```python
from build123d import *

# Parameters (mm, degrees)
SKETCH1_R                         = 5
BOSS_EXTRUDE1_DEPTH               = 2
SKETCH2_W                         = 2
SKETCH2_H                         = 4
CUT_EXTRUDE_THIN1_DEPTH           = 2
CUT_EXTRUDE_THIN1_DRAFT           = -17
SKETCH2_W_2                       = 4
SKETCH2_H_2                       = 2
CUT_EXTRUDE_THIN1_PROFILE_2_DEPTH = 2
CUT_EXTRUDE_THIN1_PROFILE_2_DRAFT = -17
SKETCH3_R                         = 2
BOSS_EXTRUDE2_DEPTH               = 40


with BuildPart() as part:
    # Sketch1 → Boss-Extrude1 (new body)
    with BuildSketch(Plane(origin=(0, 0, 0), x_dir=(1, 0, 0), z_dir=(0, 1, 0))):
        with Locations(Location((0, 0, 0), (0, 0, 270))):
            Circle(SKETCH1_R)
    extrude(amount=BOSS_EXTRUDE1_DEPTH)


with BuildPart() as cut_extrude_thin1_tool:
    # Sketch2 → Cut-Extrude-Thin1 (with draft: the straight prism first)
    with BuildSketch(Plane(origin=(0, 2, 0), x_dir=(1, 0, 0), z_dir=(0, 1, 0))):
        Rectangle(SKETCH2_W, SKETCH2_H)
    extrude(amount=-CUT_EXTRUDE_THIN1_DEPTH)
    # Cut-Extrude-Thin1: the draft: its side faces are tilted about the plane it starts from
    cut_extrude_thin1_sides = [cut_extrude_thin1_tool.faces().sort_by_distance(p)[0] for p in [
        (1, 1, 0),
        (0, 1, -2),
        (-1, 1, 0),
        (0, 1, 2),
    ]]
    draft(cut_extrude_thin1_sides, Plane(origin=(0, 2, 0), x_dir=(1, 0, 0), z_dir=(0, 1, 0)), CUT_EXTRUDE_THIN1_DRAFT)


with BuildPart() as part_1:
    add(part.part)

    # Cut-Extrude-Thin1: cut by cut_extrude_thin1_tool
    add(cut_extrude_thin1_tool.part, mode=Mode.SUBTRACT)


with BuildPart() as cut_extrude_thin1_profile_2_tool:
    # Sketch2 → Cut-Extrude-Thin1 profile 2 (with draft: the straight prism first)
    with BuildSketch(Plane(origin=(0, 2, 0), x_dir=(1, 0, 0), z_dir=(0, 1, 0))):
        Rectangle(SKETCH2_W_2, SKETCH2_H_2)
    extrude(amount=-CUT_EXTRUDE_THIN1_PROFILE_2_DEPTH)
    # Cut-Extrude-Thin1 profile 2: the draft: its side faces are tilted about the plane it starts from
    cut_extrude_thin1_profile_2_sides = [cut_extrude_thin1_profile_2_tool.faces().sort_by_distance(p)[0] for p in [
        (0, 1, 1),
        (2, 1, 0),
        (0, 1, -1),
        (-2, 1, 0),
    ]]
    draft(cut_extrude_thin1_profile_2_sides, Plane(origin=(0, 2, 0), x_dir=(1, 0, 0), z_dir=(0, 1, 0)), CUT_EXTRUDE_THIN1_PROFILE_2_DRAFT)


with BuildPart() as part_2:
    add(part_1.part)

    # Cut-Extrude-Thin1 profile 2: cut by cut_extrude_thin1_profile_2_tool
    add(cut_extrude_thin1_profile_2_tool.part, mode=Mode.SUBTRACT)

    # Sketch3 → Boss-Extrude2 (add)
    with BuildSketch(Plane.XZ):
        with Locations(Location((0, 0, 0), (0, 0, 90))):
            Circle(SKETCH3_R)
    extrude(amount=BOSS_EXTRUDE2_DEPTH)


solid = part_2.part
```
The model under review builds one solid part; all positions refer to its coordinate system, in mm. A direction names the side the tool comes from. Give positions to 0.01 mm unless a question says otherwise; leave off trailing zeros. Write each loop counter-clockwise with the first axis right and the second up, starting at its lowest first coordinate (ties: lowest second). Pieces come first, ordered by that corner, then holes. Notation, with made-up numbers: (12.25, -28.5) - (64.25, -28.5) arc R11 cw to (64.25, -20.5) - close; hole circle Ø3 at (-15, 65.25). An arc over 180 degrees is marked (long way). Answer in a Markdown table with one row per item. Add a question column.
1. Wall thickness on line 1 along Y through (x, z) = (1.5, -4.5); line 2 along Y through (x, z) = (-0.75, 0); line 3 along Z through (x, y) = (0.75, -0.5): over which ranges is each line inside the solid? List them lowest first. Write a range as [from, to].
2. Draft analysis for pull direction Z (two halves, no side actions). For faces 1 (the flat face through (1.183, 1.014, -0.699)), 2 (the cylindrical face through (2, -20, 0)), 3 (the flat face through (0.1, 0, 2.2)), state which applies: +Z half, -Z half, draft (parallel to the pull), parting line (faces both ways), or undercut.
3. We need section C-C on y = -16. Write out the cut boundary in (x, z), then the cut area to 3 significant figures.
4. Tool access review of faces 4 (the flat face through (-0.014, 1.236, -1.766)), 5 (the flat face through (1.2, 2, -1.2)): name each direction out of +Z, -Z, +X, -X, +Y, -Y from which nothing blocks a thin tool from reaching the whole face with its end or side.
5. We need section B-B on z = 0. Write out the cut boundary in (x, y).
6. Insertion check: P1, Ø6, axis at x = -1, y = -20, coming from the +Z side; P2, Ø6, axis at y = -31, z = -3, coming from the -X side; P3, Ø3, axis at x = -3.5, z = 1, coming from the -Y side. Each pin has a flat end and moves straight along its axis. Give the tip position at first contact, or say it passes through.
7. We need section D-D on z = -4. Write out the cut boundary in (x, y).
8. We need section A-A on x = 0. Write out the cut boundary in (y, z), then the cut area to 3 significant figures.
Ans:
| question | item | result |
|---|---|---|
| 1 | line 1 | y = [0, 2] |
| 1 | line 2 | y = [-40, 0] |
| 1 | line 3 | z = [-1.85, 1.85] |
| 2 | face 1 | undercut |
| 2 | face 2 | parting line |
| 2 | face 3 | draft |
| 3 | outline | circle Ø4 at (0, 0) |
| 3 | area | 12.6 mm^2 |
| 4 | face 4 | +Y |
| 4 | face 5 | +Z, -Z, +X, -X, +Y |
| 5 | outline | (-5, 0) - (-2, 0) - (-2, -40) - (2, -40) - (2, 0) - (5, 0) - (5, 2) - (2, 2) - (1.39, 0) - (-1.39, 0) - (-2, 2) - (-5, 2) - close |
| 6 | P1 | stops at z = 2 |
| 6 | P2 | stops at x = -2 |
| 6 | P3 | stops at y = 0 |
| 7 | outline | (-3, 0) - (3, 0) - (3, 2) - (-3, 2) - close |
| 8 | outline | (-40, -2) - (0, -2) - (0, -5) - (2, -5) - (2, -2) - (0, -1.39) - (0, 1.39) - (2, 2) - (2, 5) - (0, 5) - (0, 2) - (-40, 2) - close |
| 8 | area | 173 mm^2 |
